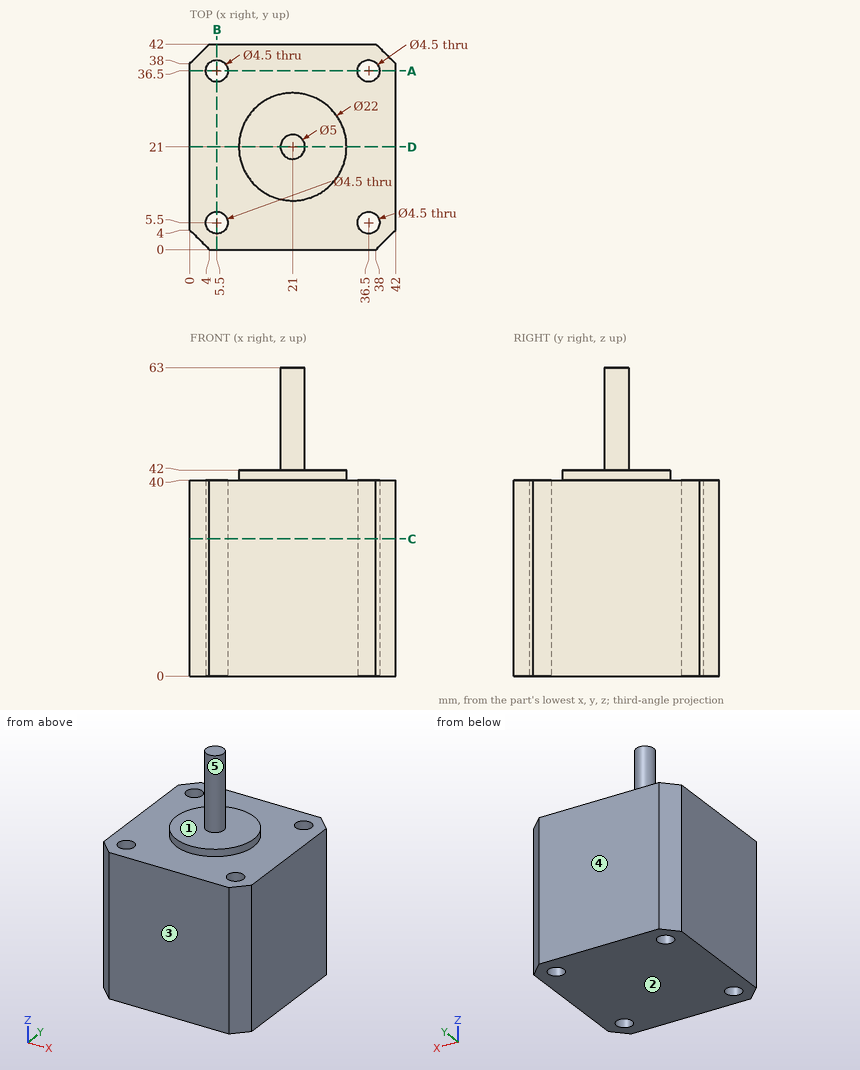
For this review, use the dimensioned drawing (mm, ordinates from the lowest corner) and the shaded views. A direction names the side the tool comes from. Round coordinates to 2 decimals unless told otherwise and drop trailing zeros. Write each loop counter-clockwise with the first axis right and the second up, starting at its lowest first coordinate (ties: lowest second). Pieces come first, ordered by that corner, then holes. Notation, with made-up numbers: M 26.5,-13.5 L 58.5,-13.5 A34 cw 58.5,20.5 Z; hole C 80,33 d11. An arc over 180 degrees is marked long. Answer as CSV lines item,"result". Start each with the question number.
Q1. Tool access review of the marked faces 4 and 5: name each direction out of +Z, -Z, +X, -X, +Y, -Y from which nothing blocks a thin tool from reaching the whole face with its end or side.
Q2. Clearance check with flat-ended pins moving along their axes: P1, Ø6, axis at x = 23.5, y = 27, coming from the +Z side; P2, Ø3.5, axis at x = 36.5, y = 5.5, coming from the +Z side. State where each tip first meets the part, or that it passes through.
Q3. Consider section D-D, the plane y = 21. Give the boundary of the cut face in (x, z), then the cut area to 3 significant figures.
Q4. Consider section A-A, the plane y = 36.5. Give the boundary of the cut face in (x, z), then the cut area to 3 significant figures.
Q5. Wall thickness on line 1 along X through (y, z) = (5, 21); line 2 along Z through (x, y) = (21, 11); line 3 along X through (y, z) = (7, 6): over which ranges is each line inside the solid? List them lowest first.
Q6. The part is to be moulded in two halves that separate along Z. For the marked faces 1, 2 and 3, say which applies: +Z half, -Z half, draft (parallel to the pull), parting line (faces both ways), or undercut.
Q7. Consider section C-C, the plane z = 28. Give the boundary of the cut face in (x, y), then the cut area to 3 significant figures.
Result set:
1,face 4,"+Z, -Z, +X, -X, +Y"
1,face 5,"+Z"
2,P1,"stops at z = 42"
2,P2,"passes through"
3,outline,"M 0,0 L 42,0 L 42,40 L 32,40 L 32,42 L 23.5,42 L 23.5,63 L 18.5,63 L 18.5,42 L 10,42 L 10,40 L 0,40 Z"
3,area,"1,830 mm²"
4,outline,"M 0,0 L 3.25,0 L 3.25,40 L 0,40 Z; M 7.75,0 L 34.25,0 L 34.25,40 L 7.75,40 Z; M 38.75,0 L 42,0 L 42,40 L 38.75,40 Z"
4,area,"1,320 mm²"
5,line 1,"x = 0 to 3.31, 7.69 to 34.31, 38.69 to 42"
5,line 2,"z = 0 to 42"
5,line 3,"x = 0 to 3.82, 7.18 to 34.82, 38.18 to 42"
6,face 1,"+Z half"
6,face 2,"-Z half"
6,face 3,"draft"
7,outline,"M 0,4 L 4,0 L 38,0 L 42,4 L 42,38 L 38,42 L 4,42 L 0,38 Z; hole C 5.5,5.5 d4.5; hole C 5.5,36.5 d4.5; hole C 36.5,5.5 d4.5; hole C 36.5,36.5 d4.5"
7,area,"1,670 mm²"
